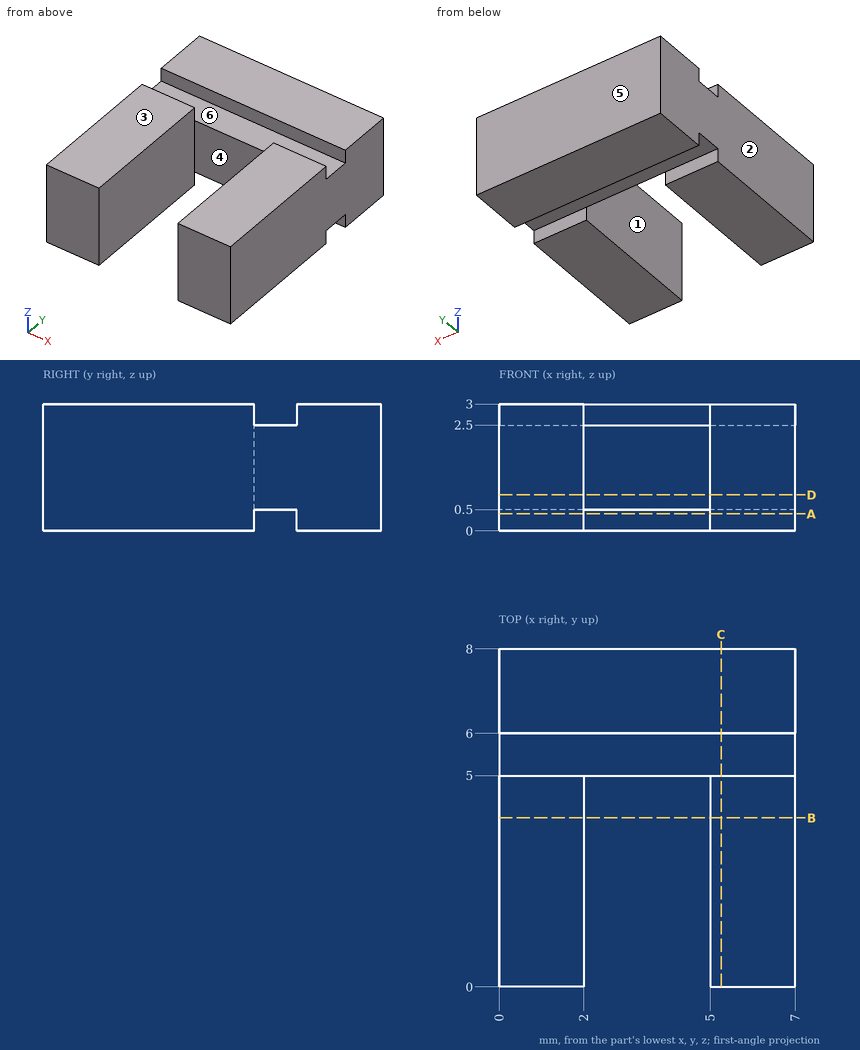
For this review, use the dimensioned drawing (mm, ordinates from the lowest corner) and the shaded views. A direction names the side the tool comes from. Give positions to 0.01 mm unless a question says otherwise; leave off trailing zeros. Loops run counter-clockwise (first coordinate to the right, second up) from the corner with the lowest first, then second, coordinate; pieces in that order, holes last.
Item 1: Take a section at A-A, the plane z = 0.4. State the section outline as (x, y) points.
Item 2: Take a section at C-C, the plane x = 5.25. State the section outline as (y, z) points.
Item 3: Take a section at B-B, the plane y = 4. State the section outline as (x, z) points, and give its area (3 significant figures).
Item 4: Draft analysis for pull direction X (two halves, no side actions). For the marked faces 1, 2 and 3, state which applies: +X half, -X half, draft (parallel to the pull), parting line (faces both ways), or undercut.
Item 5: Take a section at D-D, the plane z = 0.85. State the section outline as (x, y) points, and give its area (3 significant figures).
Item 6: Insertion check: pin 1 (0.9 mm diameter, centred on y = 3, z = 1.5, fed in from -X); pin 2 (0.6 mm diameter, centred on x = 4.5, z = 2.5, fed in from -Y); pin 3 (0.6 mm diameter, centred on x = 3.5, z = 0, fed in from -Y); pin 4 (0.8 mm diameter, centred on x = 3, y = 5.5, fed in from -Z). Each pin has a flat end and moves straight along its axis. Give the tip position at first contact, or say it passes through.
Item 7: For line 1 along X through (y, z) = (1, 2.3); line 2 along Y through (x, z) = (2.75, 0.95); line 3 along Y through (x, z) = (6.5, 0.1), list the stretches that pass through material, from the lowest coordinate up.
Item 8: Tool access review of the marked faces 4, 5 and 6: name each direction out of +Z, -Z, +X, -X, +Y, -Y from which nothing blocks a thin tool from reaching the whole face with its end or side.
Calculated:
1. outline: (0, 0) - (2, 0) - (2, 5) - (0, 5) - close; (0, 6) - (7, 6) - (7, 8) - (0, 8) - close; (5, 0) - (7, 0) - (7, 5) - (5, 5) - close
2. outline: (0, 0) - (5, 0) - (5, 0.5) - (6, 0.5) - (6, 0) - (8, 0) - (8, 3) - (6, 3) - (6, 2.5) - (5, 2.5) - (5, 3) - (0, 3) - close
3. outline: (0, 0) - (2, 0) - (2, 3) - (0, 3) - close; (5, 0) - (7, 0) - (7, 3) - (5, 3) - close
3. area: 12.0 mm2
4. face 1: undercut
4. face 2: -X half
4. face 3: draft
5. outline: (0, 0) - (2, 0) - (2, 5) - (5, 5) - (5, 0) - (7, 0) - (7, 8) - (0, 8) - close
5. area: 41.0 mm2
6. pin 1: stops at x = 0
6. pin 2: stops at y = 5
6. pin 3: stops at y = 6
6. pin 4: stops at z = 0.5
7. line 1: x = 0 to 2, 5 to 7
7. line 2: y = 5 to 8
7. line 3: y = 0 to 5, 6 to 8
8. face 4: +Z, -Z, -Y
8. face 5: +Z, -Z, +X, -X, +Y
8. face 6: +Z, +X, -X
